from build123d import *

# Parameters (mm, degrees)
SKETCH1_W           = 42
SKETCH1_H           = 42
BOSS_EXTRUDE1_DEPTH = 1
BOSS_EXTRUDE2_DEPTH = 5
FILLET1_R           = 2


with BuildPart() as part:
    # Sketch1 → Boss-Extrude1 (new body)
    with BuildSketch(Plane(origin=(0, 0, 0), x_dir=(1, 0, 0), z_dir=(0, 1, 0))):
        Rectangle(SKETCH1_W, SKETCH1_H)
        with BuildLine():
            Line((-14, -18.5), (14, -18.5))
            ThreePointArc((14, -18.5), (17.181980515, -17.181980515), (18.5, -14))
            Line((18.5, -14), (18.5, 14))
            ThreePointArc((18.5, 14), (17.181980515, 17.181980515), (14, 18.5))
            Line((14, 18.5), (-14, 18.5))
            ThreePointArc((-14, 18.5), (-17.181980515, 17.181980515), (-18.5, 14))
            Line((-18.5, 14), (-18.5, -14))
            ThreePointArc((-18.5, -14), (-17.181980515, -17.181980515), (-14, -18.5))
        make_face(mode=Mode.SUBTRACT)
    extrude(amount=BOSS_EXTRUDE1_DEPTH)

    # Sketch1<2> → Boss-Extrude2 (add)
    with BuildSketch(Plane(origin=(0, 0, 0), x_dir=(1, 0, 0), z_dir=(0, 1, 0))):
        with BuildLine():
            Line((18.5, -14), (18.5, 14))
            ThreePointArc((18.5, 14), (17.181980515, 17.181980515), (14, 18.5))
            Line((14, 18.5), (-14, 18.5))
            ThreePointArc((-14, 18.5), (-17.181980515, 17.181980515), (-18.5, 14))
            Line((-18.5, 14), (-18.5, -14))
            ThreePointArc((-18.5, -14), (-17.181980515, -17.181980515), (-14, -18.5))
            Line((-14, -18.5), (14, -18.5))
            ThreePointArc((14, -18.5), (17.181980515, -17.181980515), (18.5, -14))
        make_face()
    extrude(amount=BOSS_EXTRUDE2_DEPTH)

    # Fillet1
    fillet1_edges = [part.edges().sort_by_distance(p)[0] for p in [
        (0, 5, -18.5),
        (-18.5, 5, 0),
        (17.181980515, 5, 17.181980515),
        (18.5, 5, 0),
        (17.181980515, 5, -17.181980515),
        (-17.181980515, 5, -17.181980515),
        (-17.181980515, 5, 17.181980515),
        (0, 5, 18.5),
    ]]
    fillet(fillet1_edges, radius=FILLET1_R)


solid = part.part
Build history of the part. All positions in model axes, mm. A direction names the side the tool comes from. Coordinates: 2 decimals unless noted, no trailing zeros. Write each loop counter-clockwise with the first axis right and the second up, starting at its lowest first coordinate (ties: lowest second). Pieces come first, ordered by that corner, then holes.
(1) Cut at A-A on z = -11. List the corners of the cut face in (x, y).
(2) Cut at D-D on y = 4.05. List the corners of the cut face in (x, z).
(3) Drill centre lines: line 1 (Z direction, x = -1, y = 2.25); line 2 (X direction, y = 3.15, z = 12.5); line 3 (Y direction, x = -19, z = -9.5). Where is each one in solid material? Low to high.
(4) Cut at C-C on y = 1.55. List the corners of the cut face in (x, z), and give its area (3 significant figures).
(5) 3-axis set-ups, long thin cutter, end or side, ignore diameter. For faces 1 (the cylindrical face through (17.217, 1.986, -17.147)), 2 (the flat face through (0, 1, -19)), 3 (the flat face through (0, 2, -18.5)), 4 (the flat face through (-18.5, 2, 0)), 5 (the cylindrical face through (-17.217, 1.986, 17.147)): which of +Z, -Z, +X, -X, +Y, -Y reach the whole face in a straight line?
(6) Cut at B-B on x = 6.5. List the corners of the cut face in (y, z).
(7) Pin check, flat tips, straight feed: pin 1 Ø1.6 at (y, z) = (2, -0.5) entering from +X; pin 2 Ø1 at (x, y) = (-6.5, 2) entering from +Z; pin 3 Ø0.6 at (x, y) = (-5, 1.5) entering from -Z. Stop position of each tip, or through.
Working result:
1. outline: (-21, 0) - (21, 0) - (21, 1) - (18.5, 1) - (18.5, 3) arc R2 ccw to (16.5, 5) - (-16.5, 5) arc R2 ccw to (-18.5, 3) - (-18.5, 1) - (-21, 1) - close
2. outline: (-18.2, -14) arc R4.2 ccw to (-14, -18.2) - (14, -18.2) arc R4.2 ccw to (18.2, -14) - (18.2, 14) arc R4.2 ccw to (14, 18.2) - (-14, 18.2) arc R4.2 ccw to (-18.2, 14) - close
3. line 1: z = -18.5 to 18.5
3. line 2: x = -18.49 to 18.49
3. line 3: y = 0 to 1
4. outline: (-18.5, -14) arc R4.5 ccw to (-14, -18.5) - (14, -18.5) arc R4.5 ccw to (18.5, -14) - (18.5, 14) arc R4.5 ccw to (14, 18.5) - (-14, 18.5) arc R4.5 ccw to (-18.5, 14) - close
4. area: 1,350 mm2
5. face 1: -Z, +X, +Y
5. face 2: +Y
5. face 3: -Z, +X, -X, +Y
5. face 4: +Z, -Z, -X, +Y
5. face 5: +Z, -X, +Y
6. outline: (0, -21) - (1, -21) - (1, -18.5) - (3, -18.5) arc R2 ccw to (5, -16.5) - (5, 16.5) arc R2 ccw to (3, 18.5) - (1, 18.5) - (1, 21) - (0, 21) - close
7. pin 1: stops at x = 18.5
7. pin 2: stops at z = 18.5
7. pin 3: stops at z = -18.5
